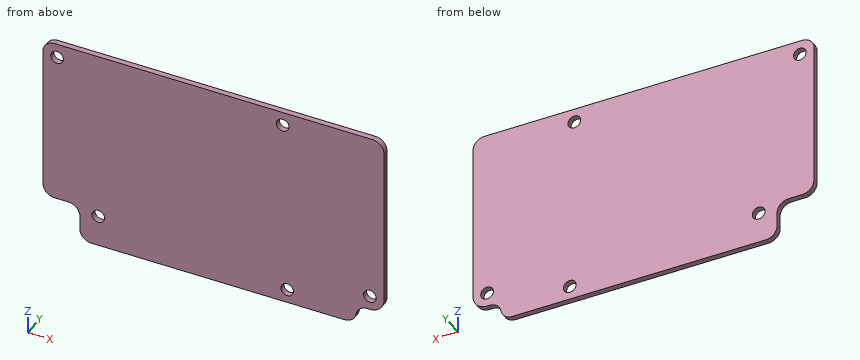
Autodesk Inventor part; units mm, degrees
ref_plane "YZ Plane" through (0, 0, 0) normal (1, 0, 0) x (0, 1, 0)
ref_plane "XZ Plane" through (0, 0, 0) normal (0, 1, 0) x (-1, 0, 0)
ref_plane "XY Plane" through (0, 0, 0) normal (0, 0, 1) x (1, 0, 0)
sketch "Sketch1" plane through (0, 0, 0) normal (0, 1, 0) x (-1, 0, 0)
  line L0 (-93.98, 0) -> (-93.98, -44.45)
  line L1 (0, -44.45) -> (0, 0)
  circle A0 centre (-15.24, -46.04) radius 1.75
  circle A1 centre (-67.3, -50.86) radius 1.75
  circle A2 centre (-66.05, -2.54) radius 1.75
  line L2 (0, -44.45) -> (-10.16, -44.45)
  line L3 (-93.98, -44.45) -> (-93.98, -54.61)
  line L4 (-93.98, -54.61) -> (-10.16, -54.61)
  line L5 (-10.16, -54.61) -> (-10.16, -44.45)
  line L6 (-66.05, 1.2192) -> (-93.98, 1.2192)
  line L7 (-93.98, 1.2192) -> (-93.98, 0)
  line L8 (-66.05, 1.2192) -> (0, 1.2192)
  line L9 (0, 1.2192) -> (0, 0)
  line L10 (0, 1.2192) -> (0, -6.5338)
  circle A3 centre (-3.8735, -2.6573) radius 1.75
  line L11 (-93.98, -49.2808) -> (-93.98, -41.5338)
  circle A4 centre (-90.1065, -45.4073) radius 1.75
extrude "Extrusion1" add sketch "Sketch1" along normal blind 1.5875
fillet "Fillet1" radius 3.175 6 edges at (0, 0.7937, 1.2192) (0, 0.7937, -44.45) (10.16, 0.7937, -44.45) (10.16, 0.7937, -54.61) (93.98, 0.7937, 1.2192) (93.98, 0.7937, -54.61)
sketch "Sketch2" plane through (0, 1.5875, 0) normal (0, 1, 0) x (1, 0, 0)
  circle A0 centre (90.1065, 45.4073) radius 1.75
  arc A1 (93.98, 45.4073) -> (90.1065, 49.2808) centre (90.1065, 45.4073) ccw
  line L0 (93.98, 1.9558) -> (93.98, 51.435)
  line L1 (86.233, 49.2808) -> (86.233, 54.61)
  line L2 (90.805, 54.61) -> (13.335, 54.61)
  line L3 (90.1065, 49.2808) -> (86.233, 49.2808)
  arc A2 (93.98, 51.435) -> (90.805, 54.61) centre (90.805, 51.435) ccw
  arc A3 (93.98, 51.435) -> (90.805, 54.61) centre (90.805, 51.435) ccw
  line L4 (93.98, 45.4073) -> (93.98, 51.435)
  line L5 (90.805, 54.61) -> (86.233, 54.61)
  point P0 (0, 0)
extrude "Extrusion2" cut sketch "Sketch2" against normal blind 25.4 contours A1 L3 L1 L2 A2 L0
fillet "Fillet2" radius 3.175 2 edges at (86.233, 0.7937, -49.2808) (86.233, 0.7937, -54.61)
properties part number "escPlate"
Input: part model. Units: mm. Frame: model coordinates. Give positions to 0.01 mm unless a question says otherwise; leave off trailing zeros. Write each loop counter-clockwise with the first axis right and the second up, starting at its lowest first coordinate (ties: lowest second). Pieces come first, ordered by that corner, then holes.
Q1. Section B-B, the plane y = 1.1. State how many separate pieces and enclosed holes the cut face has, plus the area to 3 significant figures.
Q2. Material intervals for probe 1 along Z at (x, y) = (15.24, 0.8); probe 2 along X at (y, z) = (0.65, -41.5); probe 3 along Z at (x, y) = (16.5, 1.05), sorted ascending.
Q3. First-contact query: P1, Ø4, axis at x = 3.87, z = -2.66, coming from the +Y side. Flat tip, straight axial feed; report the tip coordinate or a pass-through.
Q4. Section A-A, the plane x = 15.24. Output: boundary loops of the cut face in (y, z).
Filled in:
1. separate pieces: 1
1. enclosed holes: 5
1. area: 5,040 mm2
2. probe 1: z = -54.61 to -47.79, -44.29 to 1.22
2. probe 2: x = 0.01 to 93.98
2. probe 3: z = -54.61 to -47.25, -44.83 to 1.22
3. P1: stops at y = 1.59
4. outline: (0, -54.61) - (1.59, -54.61) - (1.59, -47.79) - (0, -47.79) - close; (0, -44.29) - (1.59, -44.29) - (1.59, 1.22) - (0, 1.22) - close
